Autodesk Inventor part; units mm, degrees
ref_plane "YZ Plane" through (0, 0, 0) normal (1, 0, 0) x (0, 1, 0)
ref_plane "XZ Plane" through (0, 0, 0) normal (0, 1, 0) x (-1, 0, 0)
ref_plane "XY Plane" through (0, 0, 0) normal (0, 0, 1) x (1, 0, 0)
sketch "Sketch1" plane through (0, 0, 0) normal (0, 0, 1) x (1, 0, 0)
  line L0 (-15, 12.5) -> (15, 12.5)
  line L1 (15, 12.5) -> (15, -12.5)
  line L2 (15, -12.5) -> (-15, -12.5)
  line L3 (-15, -12.5) -> (-15, 12.5)
  line L4 (-12, 10.5) -> (-8, 10.5)
  line L5 (-8, 10.5) -> (-8, 7.5)
  line L6 (-8, 7.5) -> (-12, 7.5)
  line L7 (-12, 7.5) -> (-12, 10.5)
  line L8 (8, 10.5) -> (12, 10.5)
  line L9 (12, 10.5) -> (12, 7.5)
  line L10 (12, 7.5) -> (8, 7.5)
  line L11 (8, 7.5) -> (8, 10.5)
  line L12 (-12, -12.5) -> (-8, -12.5)
  line L13 (-8, -12.5) -> (-8, -15.5)
  line L14 (-8, -15.5) -> (-12, -15.5)
  line L15 (-12, -15.5) -> (-12, -12.5)
  line L16 (8, -12.5) -> (12, -12.5)
  line L17 (12, -12.5) -> (12, -15.5)
  line L18 (12, -15.5) -> (8, -15.5)
  line L19 (8, -15.5) -> (8, -12.5)
  point P0 (0, 0)
  point P1 (0, 12.5)
  point P2 (15, 0)
  point P3 (-10, -12.5)
  point P4 (0, -12.5)
  point P5 (10, -12.5)
  point P6 (-10, 10.5)
  point P7 (10, 10.5)
  dimension "d0" = 25
  dimension "d1" = 30
  dimension "d2" = 4
  dimension "d3" = 3
  dimension "d4" = 3
  dimension "d5" = 4
  dimension "d6" = 10
  dimension "d7" = 10
  dimension "d8" = 10
  dimension "d9" = 10
  dimension "d10" = 20
extrude "Extrusion1" add sketch "Sketch1" along normal blind 3
properties material "MDF Medium Density Fiberboard"
Input: part model. Units: mm. Frame: model coordinates. A direction names the side the tool comes from. Give positions to 0.01 mm unless a question says otherwise; leave off trailing zeros. Order: outer loops, then holes, each group sorted by start corner. A loop starts at its lowest first (then second) coordinate and runs counter-clockwise, first axis right, second up. Notation, with made-up numbers: M -0.75,42 L 48.25,42 A22 cw 48.25,78 Z; hole C 3,0.5 d11. An arc over 180 degrees is marked long. One line per question, with ' | ' between items. Start each with the question number.
1. Access query for faces 1 (the face through (-10, 7.5, 1)), 2 (the face through (14, -12.5, 1)), 3 (the face through (0, -12.5, 1)), 4 (the face through (-13, -12.5, 1)). Directions: +Z, -Z, +X, -X, +Y, -Y. A direction counts if a zero-diameter tool reaches every point of the face in a straight line with its end or side. Return the directions, or none.
2. First-contact query: pin 1 Ø1.5 at (x, z) = (-0.5, 1.5) entering from -Y; pin 2 Ø1.5 at (y, z) = (-13.5, 1.5) entering from -X; pin 3 Ø1.5 at (y, z) = (-14.5, 2) entering from +X. Flat tips, straight axial feed; report the tip coordinate or a pass-through.
3. Section query A-A (x = 9). Return the cut outline in (y, z), and give its area (3 significant figures).
4. Material intervals for probe 1 along X at (y, z) = (8.75, 2.15); probe 2 along Y at (x, z) = (11.5, 0.6); probe 3 along X at (y, z) = (-12.75, 1.35), sorted ascending. Write a range as [from, to].
5. Pull-direction query (X, two-part tool) for faces 5 (the face through (0, -1, 3)), 6 (the face through (15, 0, 1)), 7 (the face through (-8, -14, 1)); classes: released by +X, released by -X, zero draft, split by the parting line, or undercut.
6. Section query B-B (z = 0.75). Return the cut outline in (x, y).
Here are the results:
1) face 1: +Z, -Z | face 2: +Z, -Z, +X, -Y | face 3: +Z, -Z, -Y | face 4: +Z, -Z, -X, -Y
2) pin 1: y = -12.5 | pin 2: x = -12 | pin 3: x = 12
3) outline: M -15.5,0 L 7.5,0 L 7.5,3 L -15.5,3 Z; M 10.5,0 L 12.5,0 L 12.5,3 L 10.5,3 Z | area: 75.0 mm²
4) probe 1: [-15, -12], [-8, 8], [12, 15] | probe 2: [-15.5, 7.5], [10.5, 12.5] | probe 3: [-12, -8], [8, 12]
5) face 5: zero draft | face 6: released by +X | face 7: undercut
6) outline: M -15,-12.5 L -12,-12.5 L -12,-15.5 L -8,-15.5 L -8,-12.5 L 8,-12.5 L 8,-15.5 L 12,-15.5 L 12,-12.5 L 15,-12.5 L 15,12.5 L -15,12.5 Z; hole M -12,7.5 L -8,7.5 L -8,10.5 L -12,10.5 Z; hole M 8,7.5 L 12,7.5 L 12,10.5 L 8,10.5 Z
